Drawing for the job (mm, zero at the part's lowest x, y, z). A direction names the side the tool comes from. Round coordinates to 2 decimals unless told otherwise and drop trailing zeros. Loops run counter-clockwise (first coordinate to the right, second up) from the corner with the lowest first, then second, coordinate; pieces in that order, holes last. Notation, with made-up numbers: M 74.25,32.5 L 87.25,32.5 A24 ccw 87.25,57.5 Z; hole C 77.25,62.5 d11. An arc over 180 degrees is marked long. Answer in a Markdown table with one row per item.
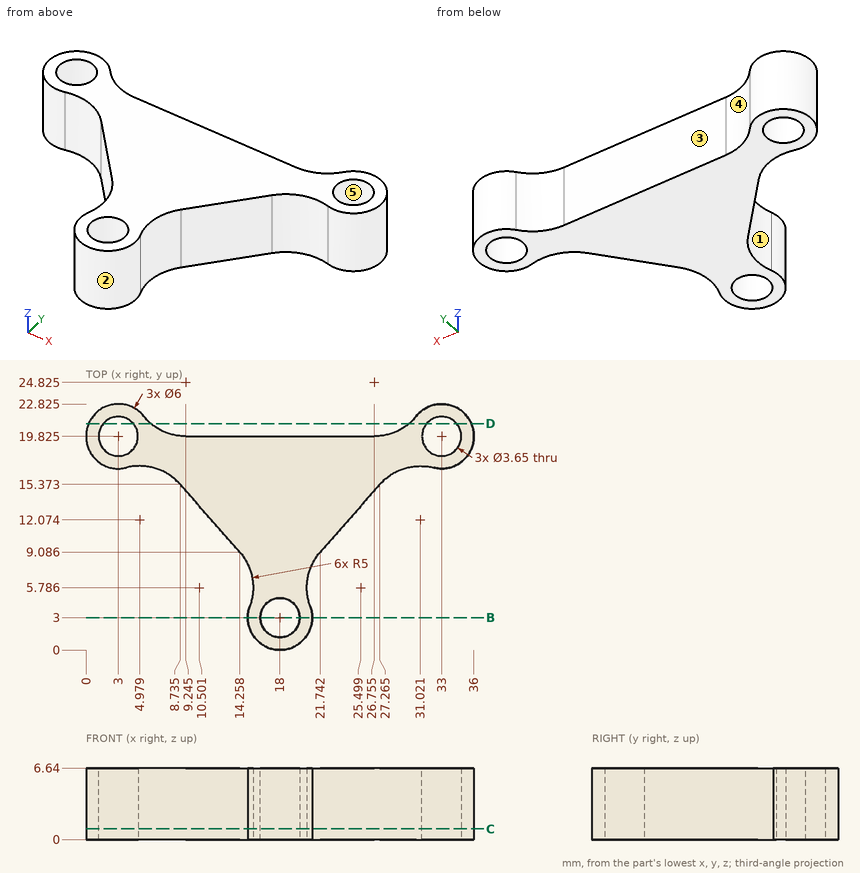
1. Wall check: probe 1 along X at (y, z) = (3, 4.5) (1 decimal); probe 2 along X at (y, z) = (21.5, 5.25) (1 decimal); probe 3 along Y at (x, z) = (18, 1.5) (1 decimal). Give the ranges that are in metal, low to high.
Verdict:
| item | result |
|---|---|
| probe 1 | x = 15 to 16.2, 19.8 to 21 |
| probe 2 | x = 0.5 to 2.3, 3.7 to 5.5, 30.5 to 32.3, 33.7 to 35.5 |
| probe 3 | y = 0 to 1.2, 4.8 to 19.8 |
2. Tool access for the marked faces 4 and 5: list every direction of +Z, -Z, +X, -X, +Y, -Y with a clear straight run to the whole face (end or side of a thin tool).
Verdict:
| item | result |
|---|---|
| face 4 | +Z, -Z, +Y |
| face 5 | +Z, -Z |
3. Mould opens along X. For the marked faces 1, 2 and 3 say: +X half, -X half, draft (parallel to the pull), parting line (faces both ways), or undercut.
Verdict:
| item | result |
|---|---|
| face 1 | -X half |
| face 2 | parting line |
| face 3 | undercut |
4. Pin check, flat tips, straight feed: pin 1 (1 mm diameter, centred on y = 8, z = 3, fed in from -X); pin 2 (2 mm diameter, centred on y = 6.5, z = 3.5, fed in from -X); pin 3 (3 mm diameter, centred on x = 23.5, z = 4, fed in from -Y). Stop position of each tip, or through.
Verdict:
| item | result |
|---|---|
| pin 1 | stops at x = 14.7 |
| pin 2 | stops at x = 15.2 |
| pin 3 | stops at y = 9.38 |
5. Saw through at B-B (y = 3). Write the cut outline in (x, z) (1 decimal), and give its area (3 significant figures).
Verdict:
| item | result |
|---|---|
| outline | M 15,0 L 16.2,0 L 16.2,6.6 L 15,6.6 Z; M 19.8,0 L 21,0 L 21,6.6 L 19.8,6.6 Z |
| area | 15.6 mm² |
6. Saw through at C-C (z = 1). State how many separate pieces and enclosed holes the cut face has.
Verdict:
| item | result |
|---|---|
| separate pieces | 1 |
| enclosed holes | 3 |
7. Saw through at D-D (y = 21). Write the cut outline in (x, z) (1 decimal).
Verdict:
| item | result |
|---|---|
| outline | M 0.2,0 L 1.6,0 L 1.6,6.6 L 0.2,6.6 Z; M 4.4,0 L 6,0 L 6,6.6 L 4.4,6.6 Z; M 30,0 L 31.6,0 L 31.6,6.6 L 30,6.6 Z; M 34.4,0 L 35.8,0 L 35.8,6.6 L 34.4,6.6 Z |
